Autodesk Inventor part; units mm, degrees
ref_plane "YZ Plane" through (0, 0, 0) normal (1, 0, 0) x (0, 1, 0)
ref_plane "XZ Plane" through (0, 0, 0) normal (0, 1, 0) x (-1, 0, 0)
ref_plane "XY Plane" through (0, 0, 0) normal (0, 0, 1) x (1, 0, 0)
sketch "Skin Scheme" plane through (0, 0, 0) normal (0, 1, 0) x (-1, 0, 0)
  line L0 (628, -84.5) -> (-628, -84.5)
  line L1 (-628, -84.5) -> (-628, 84.5)
  line L2 (-628, 84.5) -> (628, 84.5)
  line L3 (628, 84.5) -> (628, -84.5)
  circle A0 centre (506, -62.5) radius 5
  circle A1 centre (462, -62.5) radius 5
  circle A2 centre (418, -62.5) radius 5
  circle A3 centre (374, -62.5) radius 5
  circle A4 centre (330, -62.5) radius 5
  circle A5 centre (286, -62.5) radius 5
  circle A6 centre (242, -62.5) radius 5
  circle A7 centre (198, -62.5) radius 5
  circle A8 centre (154, -62.5) radius 5
  circle A9 centre (110, -62.5) radius 5
  circle A10 centre (66, -62.5) radius 5
  circle A11 centre (22, -62.5) radius 5
  circle A12 centre (-22, -62.5) radius 5
  circle A13 centre (-66, -62.5) radius 5
  circle A14 centre (-110, -62.5) radius 5
  circle A15 centre (-154, -62.5) radius 5
  circle A16 centre (-198, -62.5) radius 5
  circle A17 centre (-242, -62.5) radius 5
  circle A18 centre (506, 62.5) radius 5
  circle A19 centre (462, 62.5) radius 5
  circle A20 centre (418, 62.5) radius 5
  circle A21 centre (374, 62.5) radius 5
  circle A22 centre (330, 62.5) radius 5
  circle A23 centre (286, 62.5) radius 5
  circle A24 centre (242, 62.5) radius 5
  circle A25 centre (198, 62.5) radius 5
  circle A26 centre (154, 62.5) radius 5
  circle A27 centre (110, 62.5) radius 5
  circle A28 centre (66, 62.5) radius 5
  circle A29 centre (22, 62.5) radius 5
  circle A30 centre (-22, 62.5) radius 5
  circle A31 centre (-66, 62.5) radius 5
  circle A32 centre (-110, 62.5) radius 5
  circle A33 centre (-154, 62.5) radius 5
  circle A34 centre (-198, 62.5) radius 5
  circle A35 centre (-242, 62.5) radius 5
  circle A36 centre (-286, -62.5) radius 5
  circle A37 centre (-286, 62.5) radius 5
  circle A38 centre (-330, -62.5) radius 5
  circle A39 centre (-330, 62.5) radius 5
  circle A40 centre (-374, -62.5) radius 5
  circle A41 centre (-374, 62.5) radius 5
  circle A42 centre (-418, -62.5) radius 5
  circle A43 centre (-418, 62.5) radius 5
  circle A44 centre (-462, -62.5) radius 5
  circle A45 centre (-462, 62.5) radius 5
  circle A46 centre (-506, -62.5) radius 5
  circle A47 centre (-506, 62.5) radius 5
  point P0 (0, 0)
  dimension "d0" = 1256
  dimension "d1" = 628
  dimension "d2" = 169
  dimension "d3" = 84.5
  dimension "d4" = 10
  dimension "d5" = 122
  dimension "d6" = 22
  dimension "d9" = 44
  dimension "d12" = 125
extrude "Skin Body" add sketch "Skin Scheme" along normal blind 1
sketch "End Cut Outline" plane through (0, 1, 0) normal (0, 1, 0) x (1, 0, 0)
  line L0 (-578, 94.5) -> (-638, 94.5)
  line L1 (-638, 94.5) -> (-638, -94.5)
  line L2 (-638, -94.5) -> (-578, -94.5)
  line L3 (-578, -94.5) -> (-578, 94.5)
  line L4 (628, 84.5) -> (-628, 84.5)
  line L5 (-628, -84.5) -> (628, -84.5)
  line L6 (-628, 84.5) -> (-628, -84.5)
  point P0 (0, 0)
  dimension "d19" = 10
  dimension "d20" = 10
  dimension "d21" = 10
  dimension "d22" = 50
extrude "End Cut" cut sketch "End Cut Outline" along normal through all both and the other way through all
mirror "End Cut Mirror" about plane through (0, 0, 0) normal (1, 0, 0) of "End Cut"
properties part number "Skin NPS 10 Internal" material "Rubber, Silicone"
Here's how the part is built. I have some questions about the finished solid (model axes, mm). Give positions to 0.01 mm unless a question says otherwise; leave off trailing zeros. Use CSV: the item, a comma, the result in double quotes. Start each with the question number.
Item 1: If I drill on probe 1 along Z at (x, y) = (110, 0.6); probe 2 along Z at (x, y) = (504.5, 0.55), over which ranges is the centre line in solid material (lowest first)? Write a range as [from, to].
Item 2: I'm going to push a flat-ended pin straight in: P1, Ø9, axis at x = -242, z = 62.5, coming from the +Y side. Where does the tip first touch, or does it pass through?
Item 3: Suppose I cut it at A-A (y = 0.6). Give the number of separate pieces and of enclosed holes in the cut face, and give its area (3 significant figures).
Answer block:
1,probe 1,"z = [-84.5, -67.5], [-57.5, 57.5], [67.5, 84.5]"
1,probe 2,"z = [-84.5, -67.27], [-57.73, 57.73], [67.27, 84.5]"
2,P1,"passes through"
3,separate pieces,"1"
3,enclosed holes,"48"
3,area,"192,000 mm^2"
